Input: dimensioned drawing with shaded views. Units: mm. Origin: part minimum x, y, z. Give positions to 0.01 mm unless a question says otherwise; leave off trailing zeros. Loops run counter-clockwise (first coordinate to the right, second up) from the corner with the lowest first, then second, coordinate; pieces in that order, holes last. Notation, with made-up numbers: M -3,44.25 L 56,44.25 A6 ccw 56,52.25 Z; hole C 75,35 d6. An arc over 180 degrees is marked long. Answer in a Markdown table with one row per item.
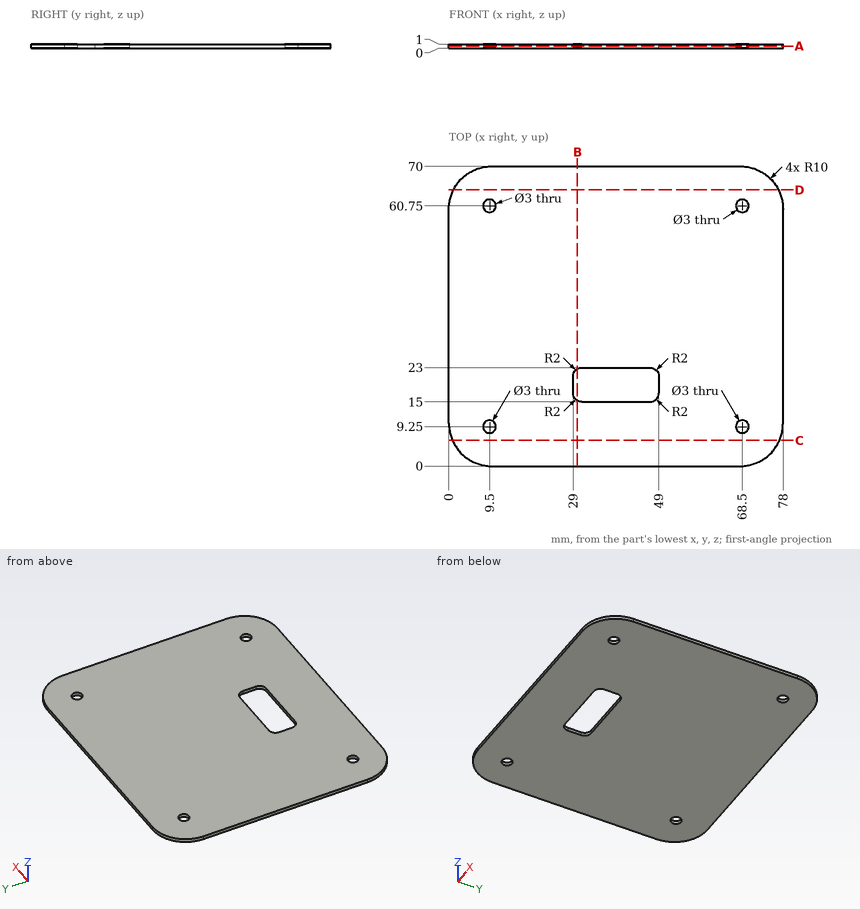
Q1. Section query B-B (x = 30). Output: boundary loops of the cut face in (y, z), plus the area to 3 significant figures.
Values follow:
| item | result |
|---|---|
| outline | M 0,0 L 15.27,0 L 15.27,1 L 0,1 Z; M 22.73,0 L 70,0 L 70,1 L 22.73,1 Z |
| area | 62.5 mm^2 |
Q2. Section query D-D (y = 64.5). Output: boundary loops of the cut face in (x, z), plus the area to 3 significant figures.
Values follow:
| item | result |
|---|---|
| outline | M 1.07,0 L 76.93,0 L 76.93,1 L 1.07,1 Z |
| area | 75.9 mm^2 |
Q3. Section query C-C (y = 6). Output: boundary loops of the cut face in (x, z).
Values follow:
| item | result |
|---|---|
| outline | M 0.83,0 L 77.17,0 L 77.17,1 L 0.83,1 Z |
Q4. Ray query, probe 1 along Y at (x, z) = (68.5, 0.6); probe 2 along Y at (x, z) = (40, 0.25); probe 3 along X at (y, z) = (8.5, 0.45). Return the intervals inside material, ascending. Write a range as from..to.
Values follow:
| item | result |
|---|---|
| probe 1 | 0.01..7.75, 10.75..59.25, 62.25..69.99 |
| probe 2 | 0..15, 23..70 |
| probe 3 | 0.11..8.2, 10.8..67.2, 69.8..77.89 |
Q5. Section query A-A (z = 0.5). Output: boundary loops of the cut face in (x, y).
Values follow:
| item | result |
|---|---|
| outline | M 0,10 A10 ccw 10,0 L 68,0 A10 ccw 78,10 L 78,60 A10 ccw 68,70 L 10,70 A10 ccw 0,60 Z; hole C 9.5,9.25 d3; hole C 9.5,60.75 d3; hole M 29,17 A2 ccw 31,15 L 47,15 A2 ccw 49,17 L 49,21 A2 ccw 47,23 L 31,23 A2 ccw 29,21 Z; hole C 68.5,9.25 d3; hole C 68.5,60.75 d3 |
